```python
from build123d import *

# Parameters (mm, degrees)
SKETCH_1_R          = 5.05
SKETCH_1_R_2        = 3.05
EXTRUDE_1_DEPTH     = 2
SKETCH_4_R          = 8
CUT_EXTRUDE_2_DEPTH = 10
CHAMFER_4_SIZE      = 10
FILLET_1_R          = 5
SKETCH_5_R          = 2
CUT_EXTRUDE_3_DEPTH = 10
SKETCH_6_R          = 1
CUT_EXTRUDE_4_DEPTH = 10
CUT_EXTRUDE_5_DEPTH = 10
CUT_EXTRUDE_6_DEPTH = 3


with BuildPart() as part:
    # 草图1 → 凸台-拉伸1 (new body)
    with BuildSketch(Plane.XY):
        with BuildLine():
            Line((-58.561307239, 85.717685223), (-68.14143119, 84.029090729))
            Line((-68.14143119, 84.029090729), (-96.085099854, 44.126897339))
            Line((-96.085099854, 44.126897339), (-78.064572289, 31.507048438))
            Line((-78.064572289, 31.507048438), (-67.064872022, 33.445857727))
            Line((-67.064872022, 33.445857727), (32.399547585, -36.209480718))
            ThreePointArc((32.399547585, -36.209480718), (61.848825623, -67.605100723), (75.145579183, -26.664396317))
            Line((75.145579183, -26.664396317), (71.375998152, -5.277939337))
            Line((71.375998152, -5.277939337), (-58.561307239, 85.717685223))
        make_face()
        with Locations((56.971703287, -54.593433609)):
            Circle(SKETCH_1_R, mode=Mode.SUBTRACT)
        with Locations((-81.097830738, 42.429451993)):
            Circle(SKETCH_1_R_2, mode=Mode.SUBTRACT)
    extrude(amount=EXTRUDE_1_DEPTH)

    # 草图4 → 切除-拉伸2 (cut)
    with BuildSketch(Plane.XY.offset(2)):
        with Locations((-61.33373119, 58.54577073)):
            Circle(SKETCH_4_R)
        with Locations((-25.29267606, 33.306072927)):
            Circle(SKETCH_4_R)
        with Locations((10.74837907, 8.066375125)):
            Circle(SKETCH_4_R)
        with Locations((46.789434199, -17.173322677)):
            Circle(SKETCH_4_R)
    extrude(amount=-CUT_EXTRUDE_2_DEPTH, mode=Mode.SUBTRACT)

    # 倒角4
    chamfer_4_edges = [part.edges().sort_by_distance(p)[0] for p in [
        (-96.085099854, 44.126897339, 1),
    ]]
    chamfer(chamfer_4_edges, length=CHAMFER_4_SIZE)

    # 圆角1
    fillet_1_edges = [part.edges().sort_by_distance(p)[0] for p in [
        (-68.14143119, 84.029090729, 1),
        (-58.561307239, 85.717685223, 1),
        (71.375998152, -5.277939337, 1),
        (32.399547585, -36.209480718, 1),
        (-67.064872022, 33.445857727, 1),
        (-78.064572289, 31.507048438, 1),
        (-87.893950961, 38.390602384, 1),
        (-90.348804899, 52.318046232, 1),
    ]]
    fillet(fillet_1_edges, radius=FILLET_1_R)

    # 草图5 → 切除-拉伸3 (cut)
    with BuildSketch(Plane(origin=(0, 0, 0), x_dir=(-1, 0, 0), z_dir=(0, 0, -1))):
        with Locations((-56.971703287, -42.593433609)):
            Circle(SKETCH_5_R)
        with Locations((-44.971703287, -54.593433609)):
            Circle(SKETCH_5_R)
        with Locations((-68.971703287, -54.593433609)):
            Circle(SKETCH_5_R)
    extrude(amount=-CUT_EXTRUDE_3_DEPTH, mode=Mode.SUBTRACT)

    # 草图6 → 切除-拉伸4 (cut)
    with BuildSketch(Plane.XY.offset(2)):
        with Locations((-52.81071672, 78.028033355)):
            Circle(SKETCH_6_R)
        with Locations((3.708210642, 38.447598165)):
            Circle(SKETCH_6_R)
        with Locations((69.237401787, -7.442761475)):
            Circle(SKETCH_6_R)
        with Locations((-44.782446967, 21.503874532)):
            Circle(SKETCH_6_R)
        with Locations((8.460020838, -15.782042676)):
            Circle(SKETCH_6_R)
    extrude(amount=-CUT_EXTRUDE_4_DEPTH, mode=Mode.SUBTRACT)

    # 草图7 → 切除-拉伸5 (cut)
    with BuildSketch(Plane(origin=(0, 0, 0), x_dir=(-1, 0, 0), z_dir=(0, 0, -1))):
        Polygon((42.900547388, 65.594166547), (11.364624149, 43.50943097), (9.643735663, 45.966775638), (41.179658901, 68.051511215), align=None)
        Polygon((-45.154303213, 3.92899578), (-13.618379974, 26.013731357), (-15.339268461, 28.471076025), (-46.875191699, 6.386340448), align=None)
    extrude(amount=-CUT_EXTRUDE_5_DEPTH, mode=Mode.SUBTRACT)

    # 草图8 → 切除-拉伸6 (cut, through all)
    with BuildSketch(Plane.XY.offset(2)):
        with BuildLine():
            Line((31.929922098, -35.060209846), (13.483519413, -22.962509091))
            Line((13.483519413, -22.962509091), (28.325536176, -95.018326982))
            Line((28.325536176, -95.018326982), (121.098918435, -54.025437146))
            Line((121.098918435, -54.025437146), (72.832718458, -13.542541133))
            Line((72.832718458, -13.542541133), (74.305789634, -29.580542184))
            ThreePointArc((74.305789634, -29.580542184), (62.030487783, -64.990252685), (34.135631, -39.96211655))
            ThreePointArc((34.135631, -39.96211655), (33.747527426, -37.189547046), (31.929922098, -35.060209846))
        make_face()
    extrude(amount=-CUT_EXTRUDE_6_DEPTH, mode=Mode.SUBTRACT)


solid = part.part
```
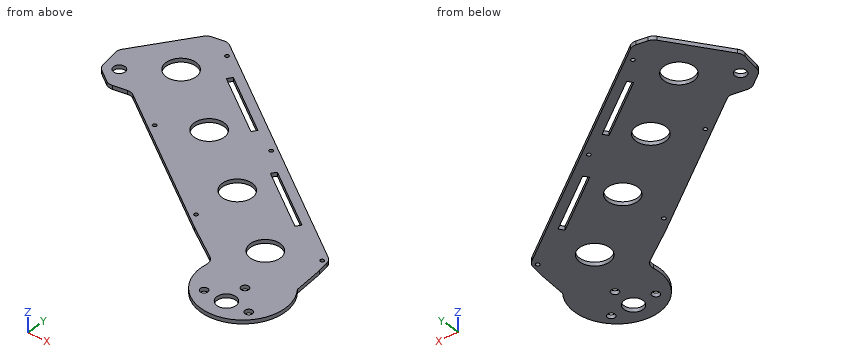
CAD build for the part. Positions are in the model's coordinates, mm. Round coordinates to 2 decimals unless told otherwise and drop trailing zeros. Order: outer loops, then holes, each group sorted by start corner. A loop starts at its lowest first (then second) coordinate and runs counter-clockwise, first axis right, second up.
Item 1: Saw through at B-B on x = 24. Write the cut outline in (y, z).
Item 2: Saw through at C-C on z = 0.9. State how many separate pieces and enclosed holes the cut face has, then the cut area to 3 significant figures.
Item 3: Pin check, flat tips, straight feed: pin 1 (10 mm diameter, centred on x = -81.1, y = 42.43, fed in from +Z); pin 2 (14.5 mm diameter, centred on x = 46.79, y = -17.17, fed in from +Z); pin 3 (1 mm diameter, centred on x = 38.5, z = 0.5, fed in from -Y). Stop position of each tip, or through.
Item 4: Saw through at A-A on y = 11. Write the cut outline in (x, z).
Item 5: Probe line 1 along X through (y, z) = (59, 0.4); line 2 along Y through (x, z) = (69, 0.85); line 3 along Y through (x, z) = (-31, 0.1). List the from-to ranges inside material, lowest first.
Reported:
1. outline: (-29.86, 0) - (18.74, 0) - (18.74, 2) - (-29.86, 2) - close; (22.41, 0) - (27.9, 0) - (27.9, 2) - (22.41, 2) - close
2. separate pieces: 1
2. enclosed holes: 16
2. area: 8,260 mm2
3. pin 1: stops at z = 2
3. pin 2: passes through
3. pin 3: stops at y = -57.47
4. outline: (-35.01, 0) - (3.31, 0) - (3.31, 2) - (-35.01, 2) - close; (18.19, 0) - (35.06, 0) - (35.06, 2) - (18.19, 2) - close; (40.29, 0) - (48.13, 0) - (48.13, 2) - (40.29, 2) - close
5. line 1: x = -85.67 to -69.32, -53.35 to -33.48, -28.25 to -20.41
5. line 2: y = -61.85 to -56.59, -52.59 to -8.41, -6.47 to -3.61
5. line 3: y = 8.19 to 27.7, 38.91 to 57.26, 60.92 to 66.42
